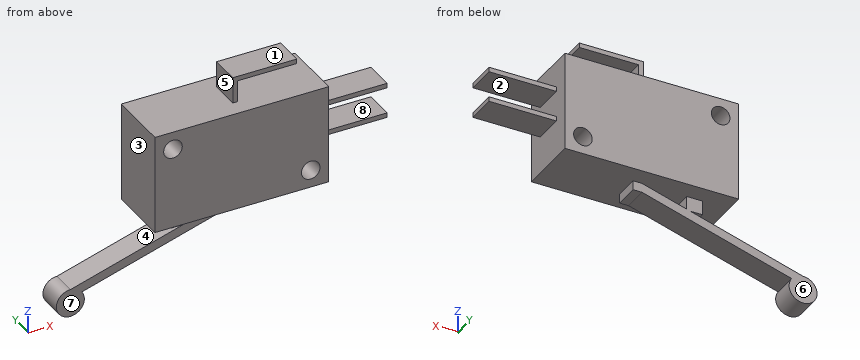
from build123d import *

# Parameters (mm, degrees)
SKETCH1_R           = 1.5
BOSS_EXTRUDE1_DEPTH = 10
BOSS_EXTRUDE2_START = 3.1
BOSS_EXTRUDE2_DEPTH = 4
BOSS_EXTRUDE3_START = 2.7
SKETCH1_4_W         = 10.85
SKETCH1_4_H         = 0.753741083
BOSS_EXTRUDE3_DEPTH = 4.8


with BuildPart() as part:
    # Sketch1 → Boss-Extrude1 (new body)
    with BuildSketch(Plane(origin=(0, 0, 0), x_dir=(1, 0, 0), z_dir=(0, 1, 0))):
        Polygon((15.43, 0), (14, 0), (6.81, 0), (4.25, 0), (0, 0), (0, -16), (14, -16), (14.75, -16), (28, -16), (28, -11.727482166), (28, -10.973741083), (28, -6.753741083), (28, -6), (28, 0), align=None)
        with Locations(Location((2.9, -13.15, 0), (0, 0, 270))):
            Circle(SKETCH1_R, mode=Mode.SUBTRACT)
        with Locations(Location((25.1, -2.85, 0), (0, 0, 270))):
            Circle(SKETCH1_R, mode=Mode.SUBTRACT)
    extrude(amount=BOSS_EXTRUDE1_DEPTH)

    # Sketch1_3 → Boss-Extrude2 (add)
    with BuildSketch(Plane(origin=(0, 0, 0), x_dir=(1, 0, 0), z_dir=(0, 1, 0)).offset(BOSS_EXTRUDE2_START)):
        with BuildLine():
            Line((6.81, 2.13344894), (14, 0))
            Line((14, 0), (15.43, 0))
            Line((15.43, 0), (15.43, 1.494165498))
            Line((15.43, 1.494165498), (14, 1.494165498))
            Line((14, 1.494165498), (-10.114002255, 8.64938004))
            ThreePointArc((-10.114002255, 8.64938004), (-12.983466277, 11.948611382), (-11.95, 7.7))
            Line((-11.95, 7.7), (6.248701299, 2.3))
            Line((6.248701299, 2.3), (4.25, 2.3))
            Line((4.25, 2.3), (4.25, 0))
            Line((4.25, 0), (6.81, 0))
            Line((6.81, 0), (6.81, 2.13344894))
        make_face()
    extrude(amount=BOSS_EXTRUDE2_DEPTH)

    # Sketch1_4 → Boss-Extrude3 (add)
    with BuildSketch(Plane(origin=(0, 0, 0), x_dir=(1, 0, 0), z_dir=(0, 1, 0)).offset(BOSS_EXTRUDE3_START)):
        Polygon((14.75, -16), (14, -16), (14, -20.25), (24.3, -20.25), (24.3, -19.5), (14.75, -19.5), align=None)
        with Locations((33.425, -11.350611625)):
            Rectangle(SKETCH1_4_W, SKETCH1_4_H)
        with Locations((33.425, -6.376870542)):
            Rectangle(SKETCH1_4_W, SKETCH1_4_H)
    extrude(amount=BOSS_EXTRUDE3_DEPTH)


solid = part.part
Source: CAD feature listing. Evaluate the final solid. Frame: model axes, mm. Face numbers are marked on the shaded views. A direction names the side the tool comes from. Give positions to 0.01 mm unless a question says otherwise; leave off trailing zeros. Order: outer loops, then holes, each group sorted by start corner. A loop starts at its lowest first (then second) coordinate and runs counter-clockwise, first axis right, second up. Notation, with made-up numbers: (-10, 79.5) -> (33, 79.5) arc R30 ccw to (33, 109.5) -> close; hole circle Ø6 at (59.5, -15). An arc over 180 degrees is marked (long way). Write item = value, one per line.
Item 1: Section query C-C (y = 1). Output: boundary loops of the cut face in (x, z), then the cut area to 3 significant figures.
Check result:
outline = (0, 0) -> (28, 0) -> (28, 16) -> (0, 16) -> close; hole circle Ø3 at (2.9, 13.15); hole circle Ø3 at (25.1, 2.85)
area = 434 mm²
Item 2: Contact query for flat-ended pins moving along their axis: pin 1 (0.6 mm diameter, centred on y = 5.5, z = -1, fed in from +X); pin 2 (4 mm diameter, centred on y = 4, z = 18.5, fed in from +X); pin 3 (0.8 mm diameter, centred on x = 35, z = 11.5, fed in from -Y). Output: stop coordinate, or through.
Check result:
pin_1 = 15.43
pin_2 = 24.3
pin_3 = 2.7
Item 3: Set-up query: the marked faces 5, 6, 7 and 8. Return all of +Z, -Z, +X, -X, +Y, -Y with unobstructed straight access to the full face (end or side cutting, diameter ignored); none if empty.
Check result:
face_5 = +Z, -X, +Y, -Y
face_6 = -Z, +X, -X, +Y
face_7 = -Z, +X, -X, -Y
face_8 = +X, +Y, -Y
Item 4: Section query B-B (x = 25.1). Output: boundary loops of the cut face in (y, z), then the cut area to 3 significant figures.
Check result:
outline = (0, 0) -> (10, 0) -> (10, 1.35) -> (0, 1.35) -> close; (0, 4.35) -> (10, 4.35) -> (10, 16) -> (0, 16) -> close
area = 130 mm²
Item 5: Section query A-A (z = 13.15). Output: boundary loops of the cut face in (x, y).
Check result:
outline = (0, 0) -> (1.4, 0) -> (1.4, 10) -> (0, 10) -> close; (4.4, 0) -> (28, 0) -> (28, 10) -> (4.4, 10) -> close
Item 6: Mould query, pull axis Z, two halves, no side actions, for the marked faces 1, 2, 3 and 4. Classes: +Z half, -Z half, draft (parallel to the pull), parting line (faces both ways), or undercut.
Check result:
face_1 = +Z half
face_2 = undercut
face_3 = draft
face_4 = undercut
Item 7: Section query D-D (y = 4). State how many separate pieces and enclosed holes the cut face has, then the cut area to 3 significant figures.
Check result:
separate_pieces = 1
enclosed_holes = 3
area = 522 mm²
Item 8: Ray query, probe 1 along X at (y, z) = (3.5, 2.85); probe 2 along X at (y, z) = (3, 13.15); probe 3 along Z at (x, y) = (3, 9.25). Return the intervals inside material, ascending.
Check result:
probe_1 = 0 to 23.6, 26.6 to 28
probe_2 = 0 to 1.4, 4.4 to 28
probe_3 = 0 to 11.65, 14.65 to 16
